```python
from build123d import *

# Parameters (mm, degrees)
CHANFREIN1_SIZE = 0.3


with BuildPart() as part:
    # Esquisse1 → Révolution1 (revolve)
    with BuildSketch(Plane.XY):
        Polygon((12.05, 0), (12.05, 1), (6.65, 1), (6.65, 0.95), (-6.05, 0.95), (-6.05, 1), (-8.85, 1), (-8.85, 1.25), (-11.05, 1.25), (-12.05, 0.672649731), (-12.05, 0), align=None)
    revolve(axis=Axis((-12.05, 0, 0), (1, 0, 0)))

    # Chanfrein1
    chanfrein1_edges = [part.edges().sort_by_distance(p)[0] for p in [
        (12.05, -1, 0),
    ]]
    chamfer(chanfrein1_edges, length=CHANFREIN1_SIZE)


solid = part.part
```
Geometry check sheet. Reference: the model listing, model coordinates, mm. A direction names the side the tool comes from. Give positions to 0.01 mm unless a question says otherwise; leave off trailing zeros. Order: outer loops, then holes, each group sorted by start corner. A loop starts at its lowest first (then second) coordinate and runs counter-clockwise, first axis right, second up. Notation, with made-up numbers: (74, -26) - (131, -26) arc R13 cw to (131, -16) - close; hole circle Ø2 at (-8.75, 84). An arc over 180 degrees is marked (long way). Answer in a Markdown table with one row per item. Add a question column.
Q1. Material ranges on probe 1 along Z at (x, y) = (7, -0.3); probe 2 along Y at (x, z) = (6.75, 0.05); probe 3 along Y at (x, z) = (-10.75, -1.05), recorded low to high. Write a range as from..to.
Q2. Cross-section at A-A, the plane y = 0. Enter the section's corners in (x, z), then the cut area to 3 significant figures.
Q3. Cross-section at C-C, the plane x = 7.75. Enter the section's corners in (y, z).
Q4. Cross-section at D-D, the plane x = -3. Enter the section's corners in (y, z), then the cut area to 3 significant figures.
Q5. Tool access check on faces 1 (the cylindrical face through (9, 0, -1)), 2 (the cylindrical face through (0.21, -0.95, 0.04)), 3 (the flat face through (-12.05, 0, 0)). Record the directions out of +Z, -Z, +X, -X, +Y, -Y that give a thin tool (end or side, any length) a straight path to the whole face; none if there is none.
Check values:
| question | item | result |
|---|---|---|
| 1 | probe 1 | z = -0.95..0.95 |
| 1 | probe 2 | y = -1..1 |
| 1 | probe 3 | y = -0.68..0.68 |
| 2 | outline | (-12.05, -0.67) - (-11.05, -1.25) - (-8.85, -1.25) - (-8.85, -1) - (-6.05, -1) - (-6.05, -0.95) - (6.65, -0.95) - (6.65, -1) - (11.75, -1) - (12.05, -0.7) - (12.05, 0.7) - (11.75, 1) - (6.65, 1) - (6.65, 0.95) - (-6.05, 0.95) - (-6.05, 1) - (-8.85, 1) - (-8.85, 1.25) - (-11.05, 1.25) - (-12.05, 0.67) - close |
| 2 | area | 47.9 mm^2 |
| 3 | outline | circle Ø2 at (0, 0) |
| 4 | outline | circle Ø1.9 at (0, 0) |
| 4 | area | 2.84 mm^2 |
| 5 | face 1 | +X |
| 5 | face 2 | none |
| 5 | face 3 | +Z, -Z, -X, +Y, -Y |
